Can you work these out from the model? Positions are in its coordinate system, mm. A direction names the side the tool comes from. Round coordinates to 2 decimals unless told otherwise and drop trailing zeros. Order: outer loops, then holes, each group sorted by start corner. A loop starts at its lowest first (then second) coordinate and runs counter-clockwise, first axis right, second up. Notation, with made-up numbers: (6.25, 39.5) -> (52.25, 39.5) arc R12 ccw to (52.25, 43.5) -> close; hole circle Ø6 at (72.5, 51). An arc over 180 degrees is marked (long way). One line per item, written item: value.
```python
from build123d import *

# Parameters (mm, degrees)
F0_W     = 107.95
F0_H     = 107.95
F1_DEPTH = 254
F2_W     = 107.95
F2_H     = 107.95
F3_DEPTH = 254
F4_DEPTH = 107.95
F5_W     = 101.6
F5_H     = 101.6
F6_DEPTH = 203.2
F7_W     = 101.6
F7_H     = 101.6
F8_DEPTH = 203.2


with BuildPart() as f1:
    # F0 (on Top) → F1 (new body)
    with BuildSketch(Plane.XY):
        Rectangle(F0_W, F0_H)
    extrude(amount=F1_DEPTH)

    # F2 (on face) → F3 (join)
    with BuildSketch(Plane.YZ.offset(53.975)):
        with Locations((0, 200.025)):
            Rectangle(F2_W, F2_H)
    extrude(amount=F3_DEPTH)

    # F4 (add): a face of the model
    f4_faces = [f1.faces().sort_by_distance(p)[0] for p in [
        (0, 0, 0),
    ]]
    extrude(f4_faces, amount=F4_DEPTH)

    # F5 (on face) → F6 (cut)
    with BuildSketch(Plane(origin=(0, 0, -107.95), x_dir=(1, 0, 0), z_dir=(0, 0, -1))):
        Rectangle(F5_W, F5_H)
    extrude(amount=-F6_DEPTH, mode=Mode.SUBTRACT)

    # F7 (on face) → F8 (cut)
    with BuildSketch(Plane.YZ.offset(307.975)):
        with Locations((0, 200.025)):
            Rectangle(F7_W, F7_H)
    extrude(amount=-F8_DEPTH, mode=Mode.SUBTRACT)


solid = f1.part
```
Q1. I want a section at D-D on z = 219.5. List the corners of the cut face in (x, y) for me (3 decimals).
Answers below:
outline: (-53.975, -53.975) -> (307.975, -53.975) -> (307.975, -50.8) -> (104.775, -50.8) -> (104.775, 50.8) -> (307.975, 50.8) -> (307.975, 53.975) -> (-53.975, 53.975) -> close
Q2. On a 3-axis mill with a long thin cutter (end or side, diameter ignored), from which of +Z, -Z, +X, -X, +Y, -Y can I reach the whole of each face in a straight line? I mean faces 4 (the face through (-1, -50.8, -8)), 5 (the face through (208, -1, 250.825)), 6 (the face through (179, -1, 146.05)). Say none if no direction works.
Answers below:
face 4: -Z
face 5: +X
face 6: -Z, +X, +Y, -Y
Q3. We'd pull the mould along X, two halves only. Please class faces 1 (the face through (124, -1, 254)), 2 (the face through (53.975, -1, 21)), 3 (the face through (50.8, 1, -8)): released by +X, released by -X, zero draft, split by the parting line, or undercut.
Answers below:
face 1: zero draft
face 2: released by +X
face 3: undercut
Q4. I want a section at A-A on x = 261. List the corners of the cut face in (y, z) for me (3 decimals), plus the area to 3 significant figures.
Answers below:
outline: (-53.975, 146.05) -> (53.975, 146.05) -> (53.975, 254) -> (-53.975, 254) -> close; hole (-50.8, 149.225) -> (50.8, 149.225) -> (50.8, 250.825) -> (-50.8, 250.825) -> close
area: 1,330 mm^2
Q5. I want a section at C-C on y = -18.5. List the corners of the cut face in (x, z) for me (3 decimals).
Answers below:
outline: (-53.975, -107.95) -> (-50.8, -107.95) -> (-50.8, 95.25) -> (50.8, 95.25) -> (50.8, -107.95) -> (53.975, -107.95) -> (53.975, 146.05) -> (307.975, 146.05) -> (307.975, 149.225) -> (104.775, 149.225) -> (104.775, 250.825) -> (307.975, 250.825) -> (307.975, 254) -> (-53.975, 254) -> close
Q6. Will these pins go through, and if not, where does the flat tip stop? pin 1 Ø2 at (y, z) = (-7, -51) entering from +X (3 decimals); pin 2 Ø1 at (x, y) = (248.5, -19) entering from -Z.
Answers below:
pin 1: x = 53.975
pin 2: z = 146.05
Q7. Please list where these lines run through material, in increasing order: line 1 along Y through (x, z) = (226, 155) (3 decimals); line 2 along Z through (x, y) = (199, 16) (3 decimals).
Answers below:
line 1: -53.975 to -50.8, 50.8 to 53.975
line 2: 146.05 to 149.225, 250.825 to 254
Q8. I want a section at B-B on z = -75.5. List the corners of the cut face in (x, y) for me (3 decimals).
Answers below:
outline: (-53.975, -53.975) -> (53.975, -53.975) -> (53.975, 53.975) -> (-53.975, 53.975) -> close; hole (-50.8, -50.8) -> (50.8, -50.8) -> (50.8, 50.8) -> (-50.8, 50.8) -> close
